Can you work these out from the model? Positions are in its coordinate system, mm. Face numbers are marked on the shaded views. A direction names the side the tool comes from. Give positions to 0.01 mm unless a question says otherwise; leave off trailing zeros. Order: outer loops, then holes, each group sorted by start corner. A loop starts at its lowest first (then second) coordinate and runs counter-clockwise, first axis right, second up. Notation, with made-up numbers: (57.5, 55) - (111.5, 55) arc R12 cw to (111.5, 64) - close; hole circle Ø1 at (31.25, -38). An arc over 180 degrees is marked (long way). Return JSON: item names as keys, results as strings.
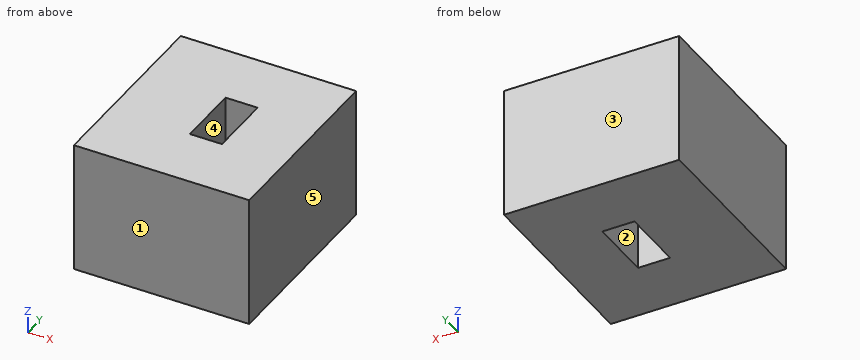
```python
from build123d import *

# Parameters (mm, degrees)
F0_W     = 25.423289
F0_H     = 27.965621
F0_W_2   = 4.660934
F0_H_2   = 9.321874
F1_DEPTH = 6.35
F2_DEPTH = 19.05


with BuildPart() as f1:
    # F0 (on Top) → F1 (new body)
    with BuildSketch(Plane.XY):
        with Locations((-37.71121, 19.279323)):
            Rectangle(F0_W, F0_H)
        with Locations((-36.440052, 19.279326)):
            Rectangle(F0_W_2, F0_H_2, mode=Mode.SUBTRACT)
    extrude(amount=F1_DEPTH)

    # F0 (on Top) → F2 (join)
    with BuildSketch(Plane.XY):
        with Locations((-37.71121, 19.279323)):
            Rectangle(F0_W, F0_H)
        with Locations((-36.440052, 19.279326)):
            Rectangle(F0_W_2, F0_H_2, mode=Mode.SUBTRACT)
    extrude(amount=F2_DEPTH)


solid = f1.part
```
1. If I drill on L1, parallel to X at y = 18.75, z = 2.75; L2, parallel to Y at x = -34.75, z = 6, over which ranges is the centre line in solid material (lowest first)? Write a range as [from, to].
Checks:
{"L1": "[-50.42, -38.77], [-34.11, -25]", "L2": "[5.3, 14.62], [23.94, 33.26]"}
2. Suppose I cut it at C-C (x = -36.25). List the corners of the cut face in (y, z) for me.
Checks:
{"outline": "(5.3, 0) - (14.62, 0) - (14.62, 19.05) - (5.3, 19.05) - close; (23.94, 0) - (33.26, 0) - (33.26, 19.05) - (23.94, 19.05) - close"}
3. Thinking about a two-plate mould opening in Y: for the marked faces 3, 4 and 5, which applies, +Y half, -Y half, draft (parallel to the pull), parting line (faces both ways), or undercut?
Checks:
{"face 3": "+Y half", "face 4": "undercut", "face 5": "draft"}
4. Suppose I cut it at A-A (y = 23). List the corners of the cut face in (x, z) for me, plus the area to 3 significant figures.
Checks:
{"outline": "(-50.42, 0) - (-38.77, 0) - (-38.77, 19.05) - (-50.42, 19.05) - close; (-34.11, 0) - (-25, 0) - (-25, 19.05) - (-34.11, 19.05) - close", "area": "396 mm^2"}
5. Suppose I cut it at B-B (z = 1.5). List the corners of the cut face in (x, y) for me, plus the area to 3 significant figures.
Checks:
{"outline": "(-50.42, 5.3) - (-25, 5.3) - (-25, 33.26) - (-50.42, 33.26) - close; hole (-38.77, 14.62) - (-34.11, 14.62) - (-34.11, 23.94) - (-38.77, 23.94) - close", "area": "668 mm^2"}
6. On a 3-axis mill with a long thin cutter (end or side, diameter ignored), from which of +Z, -Z, +X, -X, +Y, -Y can I reach the whole of each face in a straight line? I mean the marked faces 1 and 2. Say none if no direction works.
Checks:
{"face 1": "+Z, -Z, +X, -X, -Y", "face 2": "+Z, -Z"}
